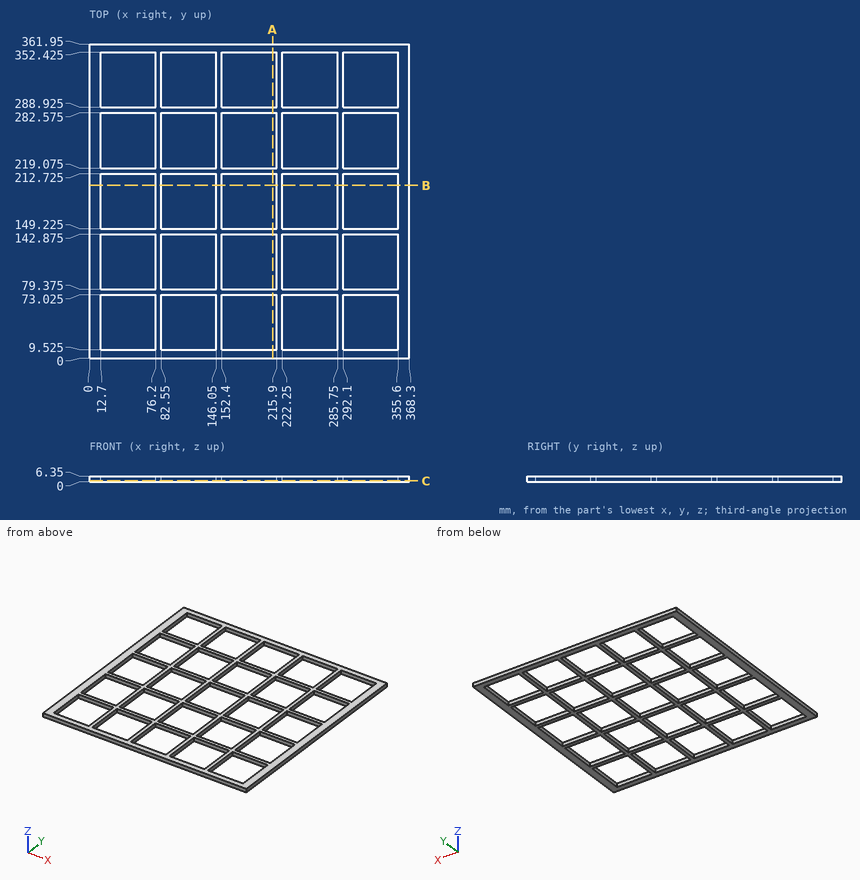
Could you check a few things on this drawing? It's one solid part, dimensions in mm from its lowest x, y, z. Round coordinates to 2 decimals unless told otherwise and drop trailing zeros. Order: outer loops, then holes, each group sorted by start corner. A loop starts at its lowest first (then second) coordinate and runs counter-clockwise, first axis right, second up. Notation, with made-up numbers: M 42.5,71 L 95.5,71 A25 cw 95.5,90 Z; hole C 29,75 d2. An arc over 180 degrees is marked long. One line per item, written item: value.
(1) Imagine slicing it at A-A (x = 211). Write out the boundary of the cut face in (y, z) (3 decimals), and give its area (3 significant figures).
Ans:
outline: M 0,0 L 9.525,0 L 9.525,6.35 L 0,6.35 Z; M 73.025,0 L 79.375,0 L 79.375,6.35 L 73.025,6.35 Z; M 142.875,0 L 149.225,0 L 149.225,6.35 L 142.875,6.35 Z; M 212.725,0 L 219.075,0 L 219.075,6.35 L 212.725,6.35 Z; M 282.575,0 L 288.925,0 L 288.925,6.35 L 282.575,6.35 Z; M 352.425,0 L 361.95,0 L 361.95,6.35 L 352.425,6.35 Z
area: 282 mm^2
(2) Imagine slicing it at C-C (z = 1). Count the separate pieces of the cut face and the enclosed holes in it, and give its area (3 significant figures).
Ans:
separate pieces: 1
enclosed holes: 25
area: 32,500 mm^2
(3) I'm going to push flat-ended pins straight in: P1, Ø3, axis at x = 30, z = 3.5, coming from the -Y side; P2, Ø1, axis at x = 75, y = 54.5, coming from the -Z side. Where does each tip first touch, or does it pass through?
Ans:
P1: stops at y = 0
P2: passes through
(4) I need wall thicknesses on line 1 along Y through (x, z) = (153.5, 4.5) (3 decimals); line 2 along X through (y, z) = (87.5, 1.75). Which ranges of each line are inside material? Lowest first, please. Write a range as from..to.
Ans:
line 1: y = 0..9.525, 73.025..79.375, 142.875..149.225, 212.725..219.075, 282.575..288.925, 352.425..361.95
line 2: x = 0..12.7, 76.2..82.55, 146.05..152.4, 215.9..222.25, 285.75..292.1, 355.6..368.3
(5) Imagine slicing it at B-B (y = 199). Write out the boundary of the cut face in (x, z).
Ans:
outline: M 0,0 L 12.7,0 L 12.7,6.35 L 0,6.35 Z; M 76.2,0 L 82.55,0 L 82.55,6.35 L 76.2,6.35 Z; M 146.05,0 L 152.4,0 L 152.4,6.35 L 146.05,6.35 Z; M 215.9,0 L 222.25,0 L 222.25,6.35 L 215.9,6.35 Z; M 285.75,0 L 292.1,0 L 292.1,6.35 L 285.75,6.35 Z; M 355.6,0 L 368.3,0 L 368.3,6.35 L 355.6,6.35 Z
